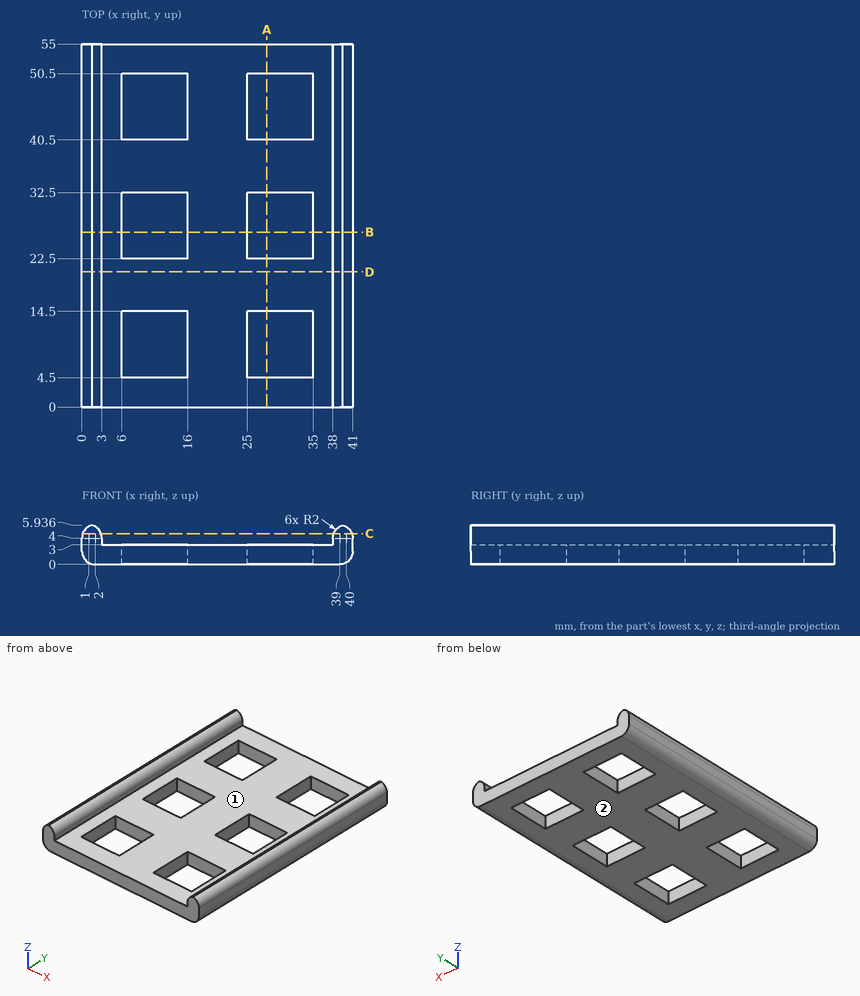
The figure shows three views and two pictorial views of one solid part (mm, origin at its lowest corner). Answer the questions. A direction names the side the tool comes from. Give positions to 0.01 mm unless a question says otherwise; leave off trailing zeros. Write each loop counter-clockwise with the first axis right and the second up, starting at its lowest first coordinate (ties: lowest second). Pieces come first, ordered by that corner, then holes.
Q1. The part is cut by section A-A on x = 28. Give the vertices of the cut face in (y, z).
Answer:
outline: (0, 0) - (4.5, 0) - (4.5, 3) - (0, 3) - close; (14.5, 0) - (22.5, 0) - (22.5, 3) - (14.5, 3) - close; (32.5, 0) - (40.5, 0) - (40.5, 3) - (32.5, 3) - close; (50.5, 0) - (55, 0) - (55, 3) - (50.5, 3) - close
Q2. Straight lines are drawn through the part: L1, parallel to Y at x = 26, z = 2; L2, parallel to X at y = 6.5, z = 3.75; L3, parallel to X at y = 23.5, z = 1.5 (1 decimal). For each, find the intervals that lie inside material, in ascending order.
Answer:
L1: y = 0 to 4.5, 14.5 to 22.5, 32.5 to 40.5, 50.5 to 55
L2: x = 0 to 3, 38 to 41
L3: x = 0.1 to 6, 16 to 25, 35 to 40.9
Q3. Given pin 1 (2 mm diameter, centred on x = 21.5, y = 49.5, fed in from +Z), flat-ended and moving along its own axis, determine where the tip first touches the part or whether it passes through.
Answer:
pin 1: stops at z = 3
Q4. The part is cut by section D-D on y = 20.5. Give the vertices of the cut face in (x, z), and give its area (3 significant figures).
Answer:
outline: (0, 2) arc R2 ccw to (2, 0) - (39, 0) arc R2 ccw to (41, 2) - (41, 4) arc R2 ccw to (39.5, 5.94) arc R2 ccw to (38, 4) - (38, 3) - (3, 3) - (3, 4) arc R2 ccw to (1.5, 5.94) arc R2 ccw to (0, 4) - close
area: 136 mm2
Q5. The part is cut by section B-B on y = 26.5. Give the vertices of the cut face in (x, z).
Answer:
outline: (0, 2) arc R2 ccw to (2, 0) - (6, 0) - (6, 3) - (3, 3) - (3, 4) arc R2 ccw to (1.5, 5.94) arc R2 ccw to (0, 4) - close; (16, 0) - (25, 0) - (25, 3) - (16, 3) - close; (35, 0) - (39, 0) arc R2 ccw to (41, 2) - (41, 4) arc R2 ccw to (39.5, 5.94) arc R2 ccw to (38, 4) - (38, 3) - (35, 3) - close
Q6. The part is cut by section C-C on z = 4.65. Give the vertices of the cut face in (x, y), and give its area (3 significant figures).
Answer:
outline: (0.11, 0) - (2.89, 0) - (2.89, 55) - (0.11, 55) - close; (38.11, 0) - (40.89, 0) - (40.89, 55) - (38.11, 55) - close
area: 306 mm2
Q7. A tool of negligible diameter and unlimited length cuts with its end or side. For the marked faces 1 and 2, from which of +Z, -Z, +X, -X, +Y, -Y can it reach the whole face along a straight path? Write none if from no direction.
Answer:
face 1: +Z, +Y, -Y
face 2: -Z, +X, -X, +Y, -Y
